Can you work these out from the drawing? Everything is in mm from the part's minimum corner. A direction names the side the tool comes from. Give positions to 0.01 mm unless a question says otherwise; leave off trailing zeros. Order: outer loops, then holes, each group sorted by start corner. A loop starts at its lowest first (then second) coordinate and runs counter-clockwise, first axis right, second up. Notation, with made-up numbers: (-17.5, -3.5) - (5.5, -3.5) arc R20 cw to (5.5, 2.5) - close; hole circle Ø10 at (19, -31.75). An arc over 180 degrees is marked (long way). One line per question, with ' | ' between items.
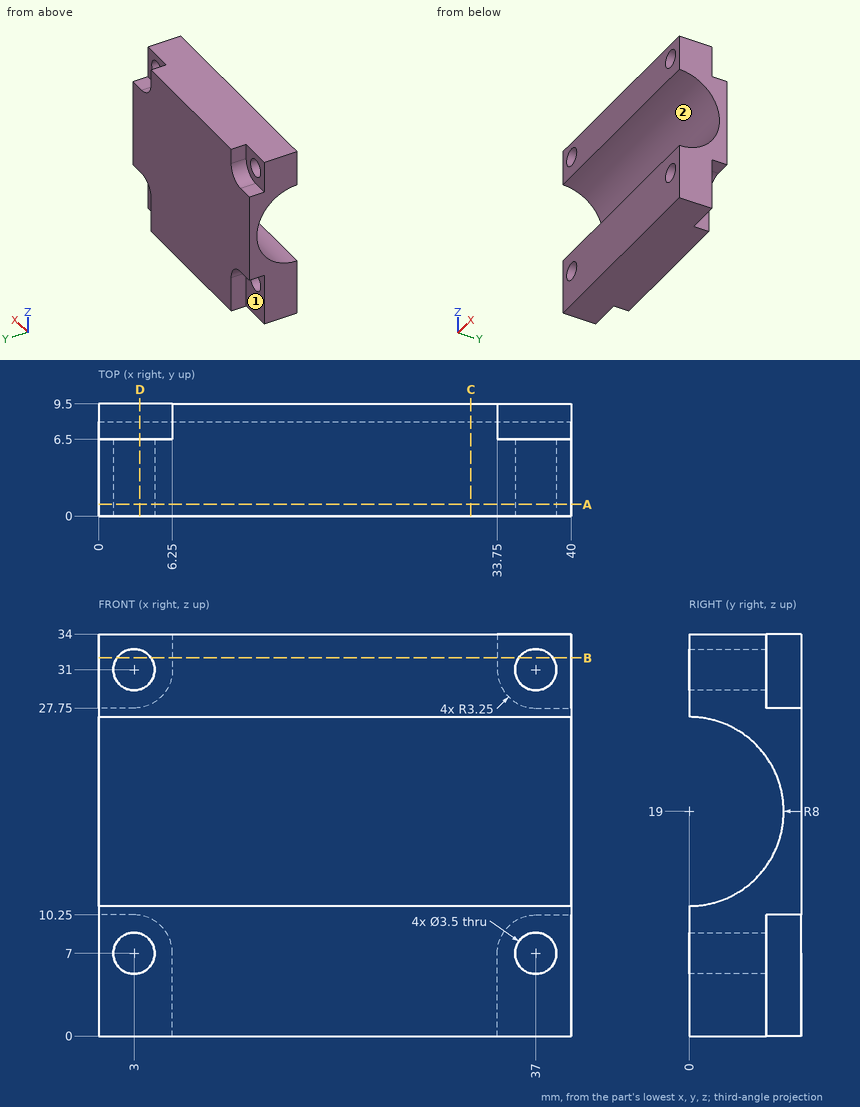
1) I want a section at A-A (y = 1). List the corners of the cut face in (x, z) for me, plus the area to 3 significant figures.
Model answer:
outline: (0, 0) - (40, 0) - (40, 11.06) - (0, 11.06) - close; (0, 26.94) - (40, 26.94) - (40, 34) - (0, 34) - close; hole circle Ø3.5 at (3, 7); hole circle Ø3.5 at (3, 31); hole circle Ø3.5 at (37, 7); hole circle Ø3.5 at (37, 31) | area: 687 mm2
2) I want a section at D-D (x = 3.5). List the corners of the cut face in (y, z) for me, plus the area to 3 significant figures.
Model answer:
outline: (0, 0) - (6.5, 0) - (6.5, 5.32) - (0, 5.32) - close; (0, 8.68) - (6.5, 8.68) - (6.5, 10.21) - (9.5, 10.21) - (9.5, 27.79) - (6.5, 27.79) - (6.5, 29.32) - (0, 29.32) - (0, 27) arc R8 cw to (0, 11) - close; (0, 32.68) - (6.5, 32.68) - (6.5, 34) - (0, 34) - close | area: 130 mm2
3) On a 3-axis mill with a long thin cutter (end or side, diameter ignored), from which of +Z, -Z, +X, -X, +Y, -Y can I reach the whole of each face in a straight line? I mean the marked faces 1 and 2. Say none if no direction works.
Model answer:
face 1: -Z, -X, +Y | face 2: +X, -X, -Y
4) Please list where these lines run through material, in increasing order: L1, parallel to X at y = 5, z = 7; L2, parallel to Z at x = 37, y = 2.25; L3, parallel to Z at x = 3, y = 1.5.
Model answer:
L1: x = 0 to 1.25, 4.75 to 35.25, 38.75 to 40 | L2: z = 0 to 5.25, 8.75 to 11.32, 26.68 to 29.25, 32.75 to 34 | L3: z = 0 to 5.25, 8.75 to 11.14, 26.86 to 29.25, 32.75 to 34
5) I want a section at C-C (x = 31.5). List the corners of the cut face in (y, z) for me.
Model answer:
outline: (0, 0) - (9.5, 0) - (9.5, 34) - (0, 34) - (0, 27) arc R8 cw to (0, 11) - close
6) I want a section at B-B (z = 32). List the corners of the cut face in (x, y) for me, plus the area to 3 significant figures.
Model answer:
outline: (0, 0) - (1.56, 0) - (1.56, 6.5) - (0, 6.5) - close; (4.44, 0) - (35.56, 0) - (35.56, 6.5) - (33.75, 6.5) - (33.75, 9.5) - (6.25, 9.5) - (6.25, 6.5) - (4.44, 6.5) - close; (38.44, 0) - (40, 0) - (40, 6.5) - (38.44, 6.5) - close | area: 305 mm2
7) I'm going to push flat-ended pins straight in: P1, Ø0.9, axis at y = 8, z = 3.5, coming from the +X side; P2, Ø7, axis at x = 37.5, z = 30, coming from the +Y side; P3, Ø1.5, axis at y = 8.5, z = 32, coming from the -X side; P4, Ø7, axis at x = 2, z = 4.5, coming from the +Y side. Where does each tip first touch, or does it pass through?
Model answer:
P1: stops at x = 33.75 | P2: stops at y = 9.5 | P3: stops at x = 6.25 | P4: stops at y = 6.5
